Design review of the part built by this model. Coordinates are the model's own, in mm. A direction names the side the tool comes from. Coordinates: 2 decimals unless noted, no trailing zeros. Loops run counter-clockwise (first coordinate to the right, second up) from the corner with the lowest first, then second, coordinate; pieces in that order, holes last. Notation, with made-up numbers: (63.5, 36) -> (105.5, 36) arc R17 cw to (105.5, 44) -> close; hole circle Ø11 at (39, 20). An arc over 180 degrees is marked (long way). Use CSV: the item, a comma, the result in double quotes.
```python
from build123d import *

# Parameters (mm, degrees)
SKETCH1_R             = 14.6812
SKETCH1_R_2           = 11.5062
BEARING_EXTRUDE_DEPTH = 4.7625
BOSS_EXTRUDE2_DEPTH   = 3.175


with BuildPart() as part:
    # Sketch1 → Bearing extrude (new, symmetric)
    with BuildSketch(Plane(origin=(0, 0, 0), x_dir=(1, 0, 0), z_dir=(0, 1, 0))):
        with Locations(Location((0, 0, 0), (0, 0, 90))):
            Circle(SKETCH1_R)
        with Locations(Location((0, 0, 0), (0, 0, 90))):
            Circle(SKETCH1_R_2, mode=Mode.SUBTRACT)
    extrude(amount=BEARING_EXTRUDE_DEPTH, both=True)

    # Sketch1_5 → Boss-Extrude2 (add, symmetric)
    with BuildSketch(Plane(origin=(0, 0, 0), x_dir=(1, 0, 0), z_dir=(0, 1, 0))):
        with BuildLine():
            Line((-7.9375, -12.350454534), (-7.9375, -55.3212))
            Line((-7.9375, -55.3212), (7.9375, -55.3212))
            Line((7.9375, -55.3212), (7.9375, -99.7712))
            Line((7.9375, -99.7712), (44.936648924, -89.431503617))
            Line((44.936648924, -89.431503617), (21.89252839, -51.421360118))
            Line((21.89252839, -51.421360118), (28.680054014, -47.306338594))
            Line((28.680054014, -47.306338594), (35.467579639, -43.19131707))
            Line((35.467579639, -43.19131707), (13.190345938, -6.446115688))
            ThreePointArc((13.190345938, -6.446115688), (3.951379748, -14.13945655), (-7.9375, -12.350454534))
        make_face()
        with BuildLine():
            ThreePointArc((3.1115, -47.3837), (0, -50.4952), (-3.1115, -47.3837))
            Line((-3.1115, -47.3837), (-3.1115, -25.4127))
            ThreePointArc((-3.1115, -25.4127), (0, -22.3012), (3.1115, -25.4127))
            Line((3.1115, -25.4127), (3.1115, -47.3837))
        make_face(mode=Mode.SUBTRACT)
        with BuildLine():
            ThreePointArc((27.225742535, -38.905724532), (27.587064378, -41.259593312), (26.178120928, -43.179523014))
            ThreePointArc((26.178120928, -43.179523014), (23.824252147, -43.540844858), (21.904322445, -42.131901407))
            Line((21.904322445, -42.131901407), (10.513942867, -23.344030478))
            ThreePointArc((10.513942867, -23.344030478), (11.561564474, -19.070231995), (15.835362956, -20.117853603))
            Line((15.835362956, -20.117853603), (27.225742535, -38.905724532))
        make_face(mode=Mode.SUBTRACT)
    extrude(amount=BOSS_EXTRUDE2_DEPTH, both=True)


solid = part.part
```
Item 1: Clearance check with flat-ended pins moving along their axes: pin 1 (1.9 mm diameter, centred on x = 0.5, y = -1.5, fed in from +Z); pin 2 (6 mm diameter, centred on x = 37, z = 72.5, fed in from +Y) (3 decimals); pin 3 (10 mm diameter, centred on x = 10.5, z = 47.5, fed in from -Y) (3 decimals). State where each tip first meets the part, or that it passes through.
Checked values:
pin 1,"z = 55.32"
pin 2,"y = 3.175"
pin 3,"y = -3.175"
Item 2: Add section B-B (x = 0). Give the boundary of the cut face in (y, z) (1 decimal), then the cut area to 3 significant figures.
Checked values:
outline,"(-4.8, -14.7) -> (4.8, -14.7) -> (4.8, -11.5) -> (-4.8, -11.5) -> close; (-4.8, 11.5) -> (4.8, 11.5) -> (4.8, 14.7) -> (3.2, 14.7) -> (3.2, 22.3) -> (-3.2, 22.3) -> (-3.2, 14.7) -> (-4.8, 14.7) -> close; (-3.2, 50.5) -> (3.2, 50.5) -> (3.2, 55.3) -> (-3.2, 55.3) -> close"
area,"140 mm^2"
Item 3: Add section D-D (z = 32.5). Give the boundary of the cut face in (x, y) (1 decimal), then the cut area to 3 significant figures.
Checked values:
outline,"(-7.9, -3.2) -> (-3.1, -3.2) -> (-3.1, 3.2) -> (-7.9, 3.2) -> close; (3.1, -3.2) -> (16.1, -3.2) -> (16.1, 3.2) -> (3.1, 3.2) -> close; (23.3, -3.2) -> (29, -3.2) -> (29, 3.2) -> (23.3, 3.2) -> close"
area,"149 mm^2"
Item 4: To check wall thickness, follow line 1 along X through (y, z) = (-0.75, 0); line 2 along X through (y, z) = (-1.75, 33); line 3 along Z through (x, y) = (34, 2.25). State the ranges of each line that lie inside material, in increasing order.
Checked values:
line 1,"-14.68 to -11.51, 11.51 to 14.68"
line 2,"-7.94 to -3.11, 3.11 to 16.37, 23.65 to 29.29"
line 3,"40.77 to 44.08, 71.39 to 92.49"
Item 5: Machinability: for faces 1 (the face through (33.576, 0.044, 70.693)), 2 (the face through (-7.938, 0, 34)), 3 (the face through (26.178, 0.044, 94.674)), 4 (the face through (0.068, 0.044, 50.494)), 5 (the face through (8, -4.762, 9)), which of the approach directions +Z, -Z, +X, -X, +Y, -Y give a long, thin tool a straight path to every point of the face, cutting with its end or side? Answer none if there is none.
Checked values:
face 1,"+X, +Y, -Y"
face 2,"+Z, -X, +Y, -Y"
face 3,"+Z, +X, +Y, -Y"
face 4,"+Y, -Y"
face 5,"+Z, -Z, +X, -X, -Y"
Item 6: Draft analysis for pull direction X (two halves, no side actions). For faces 6 (the face through (-4.41, 0.067, -14.003)), 7 (the face through (12, 3.175, 52)), 8 (the face through (-3.112, 0, 37)), state which applies: pulls with the +X half, pulls with the -X half, needs draft (parallel to the pull), parting line crosses it, or undercut.
Checked values:
face 6,"parting line crosses it"
face 7,"needs draft"
face 8,"undercut"
Item 7: Add section C-C (y = 1.75). Give the boundary of the cut face in (x, z), then the cut area to 3 significant figures.
Checked values:
outline,"(-7.94, 12.35) arc R14.68 ccw (long way) to (13.19, 6.45) -> (35.47, 43.19) -> (21.89, 51.42) -> (44.94, 89.43) -> (7.94, 99.77) -> (7.94, 55.32) -> (-7.94, 55.32) -> close; hole circle Ø23.01 at (0, 0); hole (-3.11, 25.41) arc R3.11 ccw to (3.11, 25.41) -> (3.11, 47.38) arc R3.11 ccw to (-3.11, 47.38) -> close; hole (10.51, 23.34) arc R3.11 ccw to (15.84, 20.12) -> (27.23, 38.91) arc R3.11 ccw to (21.9, 42.13) -> close"
area,"2,500 mm^2"
Item 8: Add section A-A (z = 0). Give the boundary of the cut face in (x, y).
Checked values:
outline,"(-14.68, -4.76) -> (-11.51, -4.76) -> (-11.51, 4.76) -> (-14.68, 4.76) -> close; (11.51, -4.76) -> (14.68, -4.76) -> (14.68, 4.76) -> (11.51, 4.76) -> close"
